Input: part model. Units: mm. Frame: model coordinates. Coordinates: 2 decimals unless noted, no trailing zeros. Write each loop counter-clockwise with the first axis right and the second up, starting at its lowest first coordinate (ties: lowest second). Pieces come first, ordered by that corner, then holes. Notation, with made-up numbers: (-34.5, -0.5) - (-29.5, -0.5) arc R16 ccw to (-29.5, 14.5) - close; hole circle Ø5 at (-30.5, -39.5). An arc over 180 degrees is marked (long way). Put each result on its own line as item: value. Start each with the question number.
1. Cut plane A-A, the plane z = 7. Return loops of the section in (x, y), and give its area (3 significant figures).
2. Cut plane B-B, the plane x = -659.5. Return loops of the section in (y, z), and give its area (3 significant figures).
3. Pin query (flat end, axial travel): pin 1 (1.5 mm diameter, centred on x = -196, y = 11, fed in from +Z); pin 2 (9.5 mm diameter, centred on y = 32, z = 13.5, fed in from +X). Return the tip coordinate at first contact, or that it passes through.
4. Line query: line 1 (Y direction, x = -289, z = 4); line 2 (Z direction, x = 119.5, y = 28); line 3 (X direction, y = 32.5, z = 31). Output: solid intervals per line, ascending.
5. Pull-direction query (Y, two-part tool) for faces 1 (the flat face through (10, 37, 19)), 2 (the flat face through (9, 40, 19)), 3 (the flat face through (9, -40, 19)), 4 (the flat face through (-10, -37, 19)); classes: released by +Y, released by -Y, zero draft, split by the parting line, or undercut.
from build123d import *

# Parameters (mm, degrees)
SKETCH_1_W                         = 1500
SKETCH_1_H                         = 80
SM_BASE_FLANGE_1_DEPTH             = 3
SM_EDGE_FLANGE_1_STRIP_W           = 13.4732
SM_EDGE_FLANGE_1_STRIP_H           = 3
SM_EDGE_FLANGE_1_STRIP_CUT_DEPTH   = 1500
SM_EDGE_FLANGE_1_STRIP_2_W         = 13.4732
SM_EDGE_FLANGE_1_STRIP_2_H         = 3
SM_EDGE_FLANGE_1_STRIP_CUT_2_DEPTH = 1500
SM_EDGE_FLANGE_1_DEPTH             = 1500
SM_EDGE_FLANGE_1_BEND_DEPTH        = 1500
EXTRUDE_1_DEPTH                    = 3
SKETCH_13_W                        = 74
SKETCH_13_H                        = 50
CUT_EXTRUDE_3_DEPTH                = 3
FILLET_1_R                         = 10
HOLE_WIZARD_1_AT_2_COUNT           = 2
HOLE_WIZARD_1_AT_2_PITCH           = 40
PATTERN_LINEAR_1_COUNT             = 4
PATTERN_LINEAR_1_PITCH             = 230
PATTERN_LINEAR_1_COL_COUNT         = 4
PATTERN_LINEAR_1_COL_PITCH         = 230


# Sheet-metal steps are written as plain solids
with BuildPart() as part:
    # Sketch 1 → 基体-法兰1 (new body)
    with BuildSketch(Plane.XY):
        Rectangle(SKETCH_1_W, SKETCH_1_H)
    extrude(amount=-SM_BASE_FLANGE_1_DEPTH)

    # 边线-法兰1 strip (across the edge) → 边线-法兰1 strip cut (cut)
    with BuildSketch(Plane(origin=(-750, -40, 0), x_dir=(0, 1, 0), z_dir=(1, 0, 0))):
        with Locations((-3, -1.5)):
            Rectangle(SM_EDGE_FLANGE_1_STRIP_W, SM_EDGE_FLANGE_1_STRIP_H)
    extrude(amount=SM_EDGE_FLANGE_1_STRIP_CUT_DEPTH, mode=Mode.SUBTRACT)

    # 边线-法兰1 strip 2 (across the edge) → 边线-法兰1 strip cut 2 (cut)
    with BuildSketch(Plane(origin=(750, 40, 0), x_dir=(0, -1, 0), z_dir=(-1, 0, 0))):
        with Locations((-3, -1.5)):
            Rectangle(SM_EDGE_FLANGE_1_STRIP_2_W, SM_EDGE_FLANGE_1_STRIP_2_H)
    extrude(amount=SM_EDGE_FLANGE_1_STRIP_CUT_2_DEPTH, mode=Mode.SUBTRACT)

    # 边线-法兰1 section (across the edge) → 边线-法兰1 (add)
    with BuildSketch(Plane(origin=(-750, -40, 0), x_dir=(0, 1, 0), z_dir=(1, 0, 0))):
        with BuildLine():
            Line((0, 0.7366), (0, 37))
            Line((0, 37), (3, 37))
            Line((3, 37), (3, 0.7366))
            ThreePointArc((3, 0.7366), (3.215745145, 0.215745145), (3.7366, 0))
            Line((3.7366, 0), (3.7366, -3))
            ThreePointArc((3.7366, -3), (1.094424801, -1.905575199), (0, 0.7366))
        make_face()
    extrude(amount=SM_EDGE_FLANGE_1_DEPTH)

    # 边线-法兰1 section 2 (across the edge) → 边线-法兰1 bend (add)
    with BuildSketch(Plane(origin=(750, 40, 0), x_dir=(0, -1, 0), z_dir=(-1, 0, 0))):
        with BuildLine():
            Line((0, 0.7366), (0, 37))
            Line((0, 37), (3, 37))
            Line((3, 37), (3, 0.7366))
            ThreePointArc((3, 0.7366), (3.215745145, 0.215745145), (3.7366, 0))
            Line((3.7366, 0), (3.7366, -3))
            ThreePointArc((3.7366, -3), (1.094424801, -1.905575199), (0, 0.7366))
        make_face()
    extrude(amount=SM_EDGE_FLANGE_1_BEND_DEPTH)

    # 草图12 → 凸台-拉伸1 (add)
    with BuildSketch(Plane.ZY.offset(750)):
        with BuildLine():
            Line((37, -40), (0.7366, -40))
            ThreePointArc((0.7366, -40), (-1.905575199, -38.905575199), (-3, -36.2634))
            Line((-3, -36.2634), (-3, 36.2634))
            ThreePointArc((-3, 36.2634), (-1.905575199, 38.905575199), (0.7366, 40))
            Line((0.7366, 40), (37, 40))
            Line((37, 40), (37, -40))
        make_face()
    extrude(amount=EXTRUDE_1_DEPTH)

    # 草图13 → 切除-拉伸3 (cut)
    with BuildSketch(Plane.ZY.offset(753)):
        with Locations((37, 0)):
            Rectangle(SKETCH_13_W, SKETCH_13_H)
    extrude(amount=-CUT_EXTRUDE_3_DEPTH, mode=Mode.SUBTRACT)

    # 圆角1
    fillet_1_edges = [part.edges().sort_by_distance(p)[0] for p in [
        (-751.5, 25, 37),
        (-751.5, -25, 37),
        (750, -38.5, 37),
        (750, 38.5, 37),
    ]]
    fillet(fillet_1_edges, radius=FILLET_1_R)

    # 草图15 → 打孔尺寸(%根据)内六角花形沉头螺钉的类型1 (revolve, cut)
    with BuildSketch(Plane(origin=(0, 20, 0), x_dir=(0, -1, 0), z_dir=(1, 0, 0))):
        Polygon((0, 0), (0, 26.482840043), (3.3, 24.5), (3.3, 3.1), (6.4, 0), align=None)
    hole_wizard_1 = revolve(axis=Axis((0, 20, 6.35), (0, 0, -1)), mode=Mode.SUBTRACT)

    # 打孔尺寸(%根据)内六角花形沉头螺钉的类型1 at 2: 打孔尺寸(%根据)内六角花形沉头螺钉的类型1 ×2
    with Locations(*[(0, -i * HOLE_WIZARD_1_AT_2_PITCH, 0) for i in range(1, HOLE_WIZARD_1_AT_2_COUNT)]):
        add(hole_wizard_1, mode=Mode.SUBTRACT)

    # 阵列(线性)1: 打孔尺寸(%根据)内六角花形沉头螺钉的类型1 ×4
    with Locations(*[(-i * PATTERN_LINEAR_1_PITCH, 0, 0) for i in range(1, PATTERN_LINEAR_1_COUNT)]):
        add(hole_wizard_1, mode=Mode.SUBTRACT)

    # 阵列(线性)1 copy 1 sketch → 阵列(线性)1 copy 1 (revolve, cut)
    with BuildSketch(Plane(origin=(-230, -20, 0), x_dir=(0, -1, 0), z_dir=(1, 0, 0))):
        Polygon((0, 0), (0, 26.482840043), (3.3, 24.5), (3.3, 3.1), (6.4, 0), align=None)
    revolve(axis=Axis((-230, -20, 6.35), (0, 0, -1)), mode=Mode.SUBTRACT)

    # 阵列(线性)1 copy 2 sketch → 阵列(线性)1 copy 2 (revolve, cut)
    with BuildSketch(Plane(origin=(-460, -20, 0), x_dir=(0, -1, 0), z_dir=(1, 0, 0))):
        Polygon((0, 0), (0, 26.482840043), (3.3, 24.5), (3.3, 3.1), (6.4, 0), align=None)
    revolve(axis=Axis((-460, -20, 6.35), (0, 0, -1)), mode=Mode.SUBTRACT)

    # 阵列(线性)1 copy 3 sketch → 阵列(线性)1 copy 3 (revolve, cut)
    with BuildSketch(Plane(origin=(-690, -20, 0), x_dir=(0, -1, 0), z_dir=(1, 0, 0))):
        Polygon((0, 0), (0, 26.482840043), (3.3, 24.5), (3.3, 3.1), (6.4, 0), align=None)
    revolve(axis=Axis((-690, -20, 6.35), (0, 0, -1)), mode=Mode.SUBTRACT)

    # 阵列(线性)1 col: 打孔尺寸(%根据)内六角花形沉头螺钉的类型1 ×4
    with Locations(*[(i * PATTERN_LINEAR_1_COL_PITCH, 0, 0) for i in range(1, PATTERN_LINEAR_1_COL_COUNT)]):
        add(hole_wizard_1, mode=Mode.SUBTRACT)

    # 阵列(线性)1 col copy 1 sketch → 阵列(线性)1 col copy 1 (revolve, cut)
    with BuildSketch(Plane(origin=(230, -20, 0), x_dir=(0, -1, 0), z_dir=(1, 0, 0))):
        Polygon((0, 0), (0, 26.482840043), (3.3, 24.5), (3.3, 3.1), (6.4, 0), align=None)
    revolve(axis=Axis((230, -20, 6.35), (0, 0, -1)), mode=Mode.SUBTRACT)

    # 阵列(线性)1 col copy 2 sketch → 阵列(线性)1 col copy 2 (revolve, cut)
    with BuildSketch(Plane(origin=(460, -20, 0), x_dir=(0, -1, 0), z_dir=(1, 0, 0))):
        Polygon((0, 0), (0, 26.482840043), (3.3, 24.5), (3.3, 3.1), (6.4, 0), align=None)
    revolve(axis=Axis((460, -20, 6.35), (0, 0, -1)), mode=Mode.SUBTRACT)

    # 阵列(线性)1 col copy 3 sketch → 阵列(线性)1 col copy 3 (revolve, cut)
    with BuildSketch(Plane(origin=(690, -20, 0), x_dir=(0, -1, 0), z_dir=(1, 0, 0))):
        Polygon((0, 0), (0, 26.482840043), (3.3, 24.5), (3.3, 3.1), (6.4, 0), align=None)
    revolve(axis=Axis((690, -20, 6.35), (0, 0, -1)), mode=Mode.SUBTRACT)


solid = part.part
Report:
1. outline: (-753, -40) - (750, -40) - (750, -37) - (-750, -37) - (-750, -25) - (-753, -25) - close; (-753, 25) - (-750, 25) - (-750, 37) - (750, 37) - (750, 40) - (-753, 40) - close
1. area: 9,090 mm^2
2. outline: (-40, 0.74) arc R3.74 ccw to (-36.26, -3) - (36.26, -3) arc R3.74 ccw to (40, 0.74) - (40, 37) - (37, 37) - (37, 0.74) arc R0.74 cw to (36.26, 0) - (-36.26, 0) arc R0.74 cw to (-37, 0.74) - (-37, 37) - (-40, 37) - close
2. area: 456 mm^2
3. pin 1: stops at z = 0
3. pin 2: stops at x = -750
4. line 1: y = -40 to -37, 37 to 40
4. line 2: z = -3 to 0
4. line 3: x = -753 to -750
5. face 1: undercut
5. face 2: released by +Y
5. face 3: released by -Y
5. face 4: undercut
